from build123d import *

# Parameters (mm, degrees)
F1_DEPTH = 76.2
F3_DEPTH = 152.4


with BuildPart() as f1:
    # F0 (on Front) → F1 (new body)
    with BuildSketch(Plane.XZ):
        Polygon((0, 50.8), (0, 0), (152.4, 0), (152.4, 38.1), (82.55, 38.1), (76.2, 50.8), (50.8, 50.8), (50.8, 38.1), (64.193791, 38.1), (64.193791, 25.4), (13.393791, 25.4), (13.393791, 38.1), (25.4, 38.1), (25.4, 50.8), align=None)
    extrude(amount=-F1_DEPTH)

    # F2 (on face) → F3 (cut)
    with BuildSketch(Plane.YZ.offset(152.4)):
        Polygon((12.7, 12.7), (25.4, 0), (50.8, 0), (63.5, 12.7), align=None)
    extrude(amount=-F3_DEPTH, mode=Mode.SUBTRACT)


solid = f1.part
Read the model definition and answer for the solid it produces. Units are mm, in the model's axes. A direction names the side the tool comes from. Round coordinates to 2 decimals unless told otherwise and drop trailing zeros. Loops run counter-clockwise (first coordinate to the right, second up) from the corner with the lowest first, then second, coordinate; pieces in that order, holes last.
Q1. Determine the mould class of faces 5 (the face through (75, 0, 20)), 6 (the face through (118, 38, 38.1)), 7 (the face through (77.3, 19, 6.4)) for opening direction Y: released by +Y, released by -Y, zero draft, split by the parting line, or undercut.
Q2. Section B-B on y = 56 is taken. Write down the section's boundary in (x, z), and give its area (3 significant figures).
Q3. Section C-C on x = 73 is taken. Write down the section's boundary in (y, z), and give its area (3 significant figures).
Q4. Consider probe 1 along X at (y, z) = (38, 28); probe 2 along Z at (x, y) = (55.5, 42.5); probe 3 along Z at (x, y) = (100, 31.5). Determine where each line is inside the solid, lowest interval first.
Q5. Which of the six approach directions +Z, -Z, +X, -X, +Y, -Y give full straight-line access (tool end or side, diameter ignored) to faces 1 (the face through (77.3, 57.1, 6.3)), 2 (the face through (13, 38, 50.8)), 3 (the face through (50.8, 38, 45)), 4 (the face through (39, 38, 25.4))?
Q6. Section A-A on z = 44 is taken. Write down the section's boundary in (x, y), and give its area (3 significant figures).
Q7. Section D-D on y = 9 is taken. Write down the section's boundary in (x, z), and give its area (3 significant figures).
Q8. This flat-tipped pin is pushed along its axis until it touches: pin 1 (9.5 mm diameter, centred on x = 21.5, y = 31.5, fed in from -Z). Where does it stop, or does it pass through?
Output:
1. face 5: released by -Y
1. face 6: zero draft
1. face 7: undercut
2. outline: (0, 0) - (152.4, 0) - (152.4, 5.2) - (0, 5.2) - close; (0, 12.7) - (152.4, 12.7) - (152.4, 38.1) - (82.55, 38.1) - (76.2, 50.8) - (50.8, 50.8) - (50.8, 38.1) - (64.19, 38.1) - (64.19, 25.4) - (13.39, 25.4) - (13.39, 38.1) - (25.4, 38.1) - (25.4, 50.8) - (0, 50.8) - close
2. area: 4,700 mm2
3. outline: (0, 0) - (25.4, 0) - (12.7, 12.7) - (63.5, 12.7) - (50.8, 0) - (76.2, 0) - (76.2, 50.8) - (0, 50.8) - close
3. area: 3,390 mm2
4. probe 1: x = 0 to 13.39, 64.19 to 152.4
4. probe 2: z = 12.7 to 25.4, 38.1 to 50.8
4. probe 3: z = 12.7 to 38.1
5. face 1: +X, -X
5. face 2: +Z, +X, -X, +Y, -Y
5. face 3: +Z, +Y, -Y
5. face 4: +Y, -Y
6. outline: (0, 0) - (25.4, 0) - (25.4, 76.2) - (0, 76.2) - close; (50.8, 0) - (79.6, 0) - (79.6, 76.2) - (50.8, 76.2) - close
6. area: 4,130 mm2
7. outline: (0, 0) - (152.4, 0) - (152.4, 38.1) - (82.55, 38.1) - (76.2, 50.8) - (50.8, 50.8) - (50.8, 38.1) - (64.19, 38.1) - (64.19, 25.4) - (13.39, 25.4) - (13.39, 38.1) - (25.4, 38.1) - (25.4, 50.8) - (0, 50.8) - close
7. area: 5,850 mm2
8. pin 1: stops at z = 12.7
